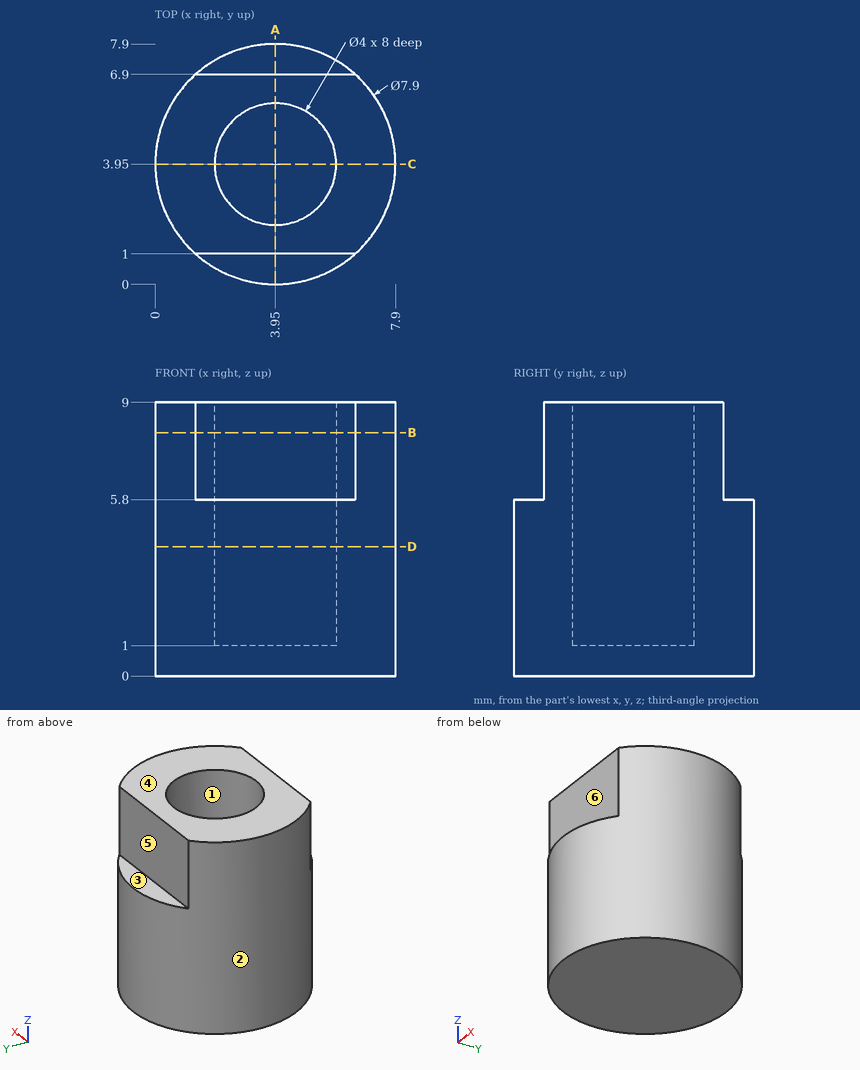
Geometry check sheet. Reference: drawing and pictorial views, mm from the part's lowest x, y, z. A direction names the side the tool comes from. Round coordinates to 2 decimals unless told otherwise and drop trailing zeros. Loops run counter-clockwise (first coordinate to the right, second up) from the corner with the lowest first, then second, coordinate; pieces in that order, holes last. Notation, with made-up numbers: (-7.75, -1) - (6.25, -1) arc R24 cw to (6.25, 18) - close; hole circle Ø4 at (-36.75, 32.25). An arc over 180 degrees is marked (long way). Write item = value, one per line. Start each with the question number.
Q1. Section check B-B (z = 8). Record the boundary of the cut face in (x, y).
Q2. Section check C-C (y = 3.95). Record the boundary of the cut face in (x, z).
Q3. Release check for a two-part mould opening along X. For the marked faces 1, 2 and 3 record: pulls with the +X half, pulls with the -X half, needs draft (parallel to the pull), parting line crosses it, or undercut.
Q4. Section check A-A (x = 3.95). Record the boundary of the cut face in (y, z).
Q5. Depth check by flat-ended pin: P1, Ø4.5, axis at x = 4.5, y = 4.5, coming from the +Z side; P2, Ø1, axis at x = 3.5, z = 6.5, coming from the -Y side; P3, Ø2.5, axis at x = 2.5, z = 8, coming from the +Y side; P4, Ø1, axis at y = 1, z = 6, coming from the -X side. Enter the tip coordinate at first touch or a pass-through.
Q6. Thickness scan on L1, parallel to Y at x = 3.95, z = 5.5; L2, parallel to Y at x = 3.95, z = 6.75; L3, parallel to Y at x = 6.25, z = 8.25. Record the ranges inside material, lowest first.
Q7. Access from +Z, -Z, +X, -X, +Y, -Y to the whole of each face (thin tool, end or side, straight path). Record for the marked faces 4, 5 and 6.
Q8. Section check D-D (z = 4.25). Record the boundary of the cut face in (x, y).
Derived:
q1.outline = (1.32, 1) - (6.58, 1) arc R3.95 ccw to (6.58, 6.9) - (1.32, 6.9) arc R3.95 ccw to start; hole circle Ø4 at (3.95, 3.95)
q2.outline = (0, 0) - (7.9, 0) - (7.9, 9) - (5.95, 9) - (5.95, 1) - (1.95, 1) - (1.95, 9) - (0, 9) - close
q3.face_1 = undercut
q3.face_2 = parting line crosses it
q3.face_3 = needs draft
q4.outline = (0, 0) - (7.9, 0) - (7.9, 5.8) - (6.9, 5.8) - (6.9, 9) - (5.95, 9) - (5.95, 1) - (1.95, 1) - (1.95, 9) - (1, 9) - (1, 5.8) - (0, 5.8) - close
q5.P1 = 9
q5.P2 = 1
q5.P3 = 6.9
q5.P4 = 0.85
q6.L1 = 0 to 1.95, 5.95 to 7.9
q6.L2 = 1 to 1.95, 5.95 to 6.9
q6.L3 = 1 to 6.9
q7.face_4 = +Z, +X, -X, +Y, -Y
q7.face_5 = +Z, +X, -X, +Y
q7.face_6 = +Z, +X, -X, -Y
q8.outline = circle Ø7.9 at (3.95, 3.95); hole circle Ø4 at (3.95, 3.95)
